Verification items for the finished model (mm, model axes). A direction names the side the tool comes from. Round coordinates to 2 decimals unless told otherwise and drop trailing zeros. Loops run counter-clockwise (first coordinate to the right, second up) from the corner with the lowest first, then second, coordinate; pieces in that order, holes last. Notation, with made-up numbers: M 9.25,28.25 L 66.25,28.25 A35 ccw 66.25,63.25 Z; hole C 67,43.5 d4. An arc over 180 degrees is marked long. One line per item, written item: value.
from build123d import *

# Parameters (mm, degrees)
SKETCH1_W          = 8
SKETCH1_H          = 8
BASE_FLANGE1_DEPTH = 0.5
EDGE_FLANGE1_DEPTH = 8
EDGE_FLANGE2_DEPTH = 8
FILLET1_R          = 4
SKETCH12_R         = 2
CUT_EXTRUDE1_DEPTH = 15.574703412
SKETCH13_R         = 2
CUT_EXTRUDE2_DEPTH = 18.548159967


# Sheet-metal steps are written as plain solids
with BuildPart() as part:
    # Sketch1 → Base-Flange1 (new body)
    with BuildSketch(Plane(origin=(0, 0, 0), x_dir=(1, 0, 0), z_dir=(0, 1, 0))):
        Rectangle(SKETCH1_W, SKETCH1_H)
    extrude(amount=BASE_FLANGE1_DEPTH)

    # Edge-Flange1 section (across the edge) → Edge-Flange1 (add)
    with BuildSketch(Plane(origin=(4.7366, 0.5, 4), x_dir=(-1, 0, 0), z_dir=(0, 0, -1))):
        with BuildLine():
            Line((-0.5, 0.7366), (-0.5, 13))
            Line((-0.5, 13), (0, 13))
            Line((0, 13), (0, 0.7366))
            ThreePointArc((0, 0.7366), (0.215745145, 0.215745145), (0.7366, 0))
            Line((0.7366, 0), (0.7366, -0.5))
            ThreePointArc((0.7366, -0.5), (-0.137808246, -0.137808246), (-0.5, 0.7366))
        make_face()
    extrude(amount=EDGE_FLANGE1_DEPTH)

    # Edge-Flange2 section (across the edge) → Edge-Flange2 (add)
    with BuildSketch(Plane(origin=(-4.7366, 0.5, -4), x_dir=(1, 0, 0), z_dir=(0, 0, 1))):
        with BuildLine():
            Line((-0.5, 0.7366), (-0.5, 13))
            Line((-0.5, 13), (0, 13))
            Line((0, 13), (0, 0.7366))
            ThreePointArc((0, 0.7366), (0.215745145, 0.215745145), (0.7366, 0))
            Line((0.7366, 0), (0.7366, -0.5))
            ThreePointArc((0.7366, -0.5), (-0.137808246, -0.137808246), (-0.5, 0.7366))
        make_face()
    extrude(amount=EDGE_FLANGE2_DEPTH)

    # Fillet1
    fillet1_edges = [part.edges().sort_by_distance(p)[0] for p in [
        (4.9866, 13.5, -4),
        (-4.9866, 13.5, -4),
        (4.9866, 13.5, 4),
        (-4.9866, 13.5, 4),
    ]]
    fillet(fillet1_edges, radius=FILLET1_R - 0.0001)  # a hair under: the kernel refuses the full size

    # Sketch12 → Cut-Extrude1 (cut, through all)
    with BuildSketch(Plane(origin=(0, 0.5, 0), x_dir=(1, 0, 0), z_dir=(0, 1, 0))):
        with Locations(Location((0, 0, 0), (0, 0, 270))):
            Circle(SKETCH12_R)
    extrude(amount=-CUT_EXTRUDE1_DEPTH, mode=Mode.SUBTRACT)

    # Sketch13 → Cut-Extrude2 (cut, through all)
    with BuildSketch(Plane(origin=(5.2366, 0, 0), x_dir=(0, 0, -1), z_dir=(1, 0, 0))):
        with Locations(Location((0, 9.484444929, 0), (0, 0, 90))):
            Circle(SKETCH13_R)
    extrude(amount=-CUT_EXTRUDE2_DEPTH, mode=Mode.SUBTRACT)


solid = part.part
(1) Depth check by flat-ended pin: pin 1 Ø3.5 at (y, z) = (9.48, 0) entering from +X; pin 2 Ø3 at (x, y) = (4, 12) entering from +Z. Enter the tip coordinate at first touch or a pass-through.
Completed:
pin 1: passes through
pin 2: stops at z = 3.82
(2) Thickness scan on L1, parallel to X at y = 6.25, z = -3; L2, parallel to Y at x = -2.5, z = -0.75. Record the ranges inside material, lowest first. Write a range as from..to.
Completed:
L1: x = -5.24..-4.74, 4.74..5.24
L2: y = 0..0.5
(3) Sectioned sample at B-B on y = 4.5. Enter the section's corners in (x, z).
Completed:
outline: M -5.24,-4 L -4.74,-4 L -4.74,4 L -5.24,4 Z; M 4.74,-4 L 5.24,-4 L 5.24,4 L 4.74,4 Z
(4) Sectioned sample at D-D on y = 8.75. Enter the section's corners in (x, z).
Completed:
outline: M -5.24,-4 L -4.74,-4 L -4.74,-1.86 L -5.24,-1.86 Z; M -5.24,1.86 L -4.74,1.86 L -4.74,4 L -5.24,4 Z; M 4.74,-4 L 5.24,-4 L 5.24,-1.86 L 4.74,-1.86 Z; M 4.74,1.86 L 5.24,1.86 L 5.24,4 L 4.74,4 Z
(5) Sectioned sample at A-A on x = 0. Enter the section's corners in (y, z), and give its area (3 significant figures).
Completed:
outline: M 0,-4 L 0.5,-4 L 0.5,-2 L 0,-2 Z; M 0,2 L 0.5,2 L 0.5,4 L 0,4 Z
area: 2.00 mm^2
(6) Tool access check on faces 1 (the face through (-4.983, 12.359, 2.797)), 2 (the face through (-4.737, 6, 0)). Record the directions out of +Z, -Z, +X, -X, +Y, -Y that give a thin tool (end or side, any length) a straight path to the whole face; none if there is none.
Completed:
face 1: +Z, +X, -X, +Y
face 2: +Z, -Z, +Y
(7) Sectioned sample at C-C on z = 1.5. Enter the section's corners in (x, y).
Completed:
outline: M -5.24,1.24 A1.24 ccw -4,0 L -1.32,0 L -1.32,0.5 L -4,0.5 A0.74 cw -4.74,1.24 L -4.74,8.16 L -5.24,8.16 Z; M -5.24,10.81 L -4.74,10.81 L -4.74,13.21 L -5.24,13.21 Z; M 1.32,0 L 4,0 A1.24 ccw 5.24,1.24 L 5.24,8.16 L 4.74,8.16 L 4.74,1.24 A0.74 cw 4,0.5 L 1.32,0.5 Z; M 4.74,10.81 L 5.24,10.81 L 5.24,13.21 L 4.74,13.21 Z
(8) Mould release check, pull along Y, two halves, no side actions. Record for faces 3 (the face through (-4.983, 12.359, -2.797)), 4 (the face through (-4.983, 7.486, 0.088)), 5 (the face through (0, 0.2, -4)): +Y half, -Y half, draft (parallel to the pull), parting line (faces both ways), or undercut.
Completed:
face 3: +Y half
face 4: undercut
face 5: draft
